Can you work these out from the model? Positions are in its coordinate system, mm. Face numbers are marked on the shaded views. A direction names the side the tool comes from. Round coordinates to 2 decimals unless told otherwise and drop trailing zeros. Loops run counter-clockwise (first coordinate to the right, second up) from the corner with the lowest first, then second, coordinate; pieces in that order, holes last. Notation, with made-up numbers: M 52.5,87 L 75.5,87 A15 ccw 75.5,116 Z; hole C 37,15.5 d11. An arc over 180 degrees is marked long. Return JSON: item names as keys, results as strings.
```python
from build123d import *

# Parameters (mm, degrees)
SKETCH_2_R      = 6.25
EXTRUDE_1_DEPTH = 15
SKETCH_3_W      = 12
SKETCH_3_H      = 18
EXTRUDE_2_DEPTH = 3
SKETCH_4_R      = 1.65
EXTRUDE_3_DEPTH = 5


with BuildPart() as part:
    # ｽｹｯﾁ2 → ﾎﾞｽ - 押し出し1 (new body)
    with BuildSketch(Plane.XY):
        Circle(SKETCH_2_R)
    extrude(amount=EXTRUDE_1_DEPTH)

    # ｽｹｯﾁ3 → ﾎﾞｽ - 押し出し2 (add)
    with BuildSketch(Plane.XY.offset(15)):
        Rectangle(SKETCH_3_W, SKETCH_3_H)
    extrude(amount=EXTRUDE_2_DEPTH)

    # ｽｹｯﾁ4 → ﾎﾞｽ - 押し出し3 (add, symmetric)
    with BuildSketch(Plane(origin=(0, 0, 0), x_dir=(0, 0, -1), z_dir=(1, 0, 0))):
        with BuildLine():
            Line((-18, 9), (-18, -9))
            Line((-18, -9), (-12, -9))
            ThreePointArc((-12, -9), (-65.69848481, 4.757359313), (-18, 33))
            Line((-18, 33), (-18, 9))
        make_face()
        with Locations((-36, 9)):
            Circle(SKETCH_4_R, mode=Mode.SUBTRACT)
    extrude(amount=EXTRUDE_3_DEPTH, both=True)


solid = part.part
```
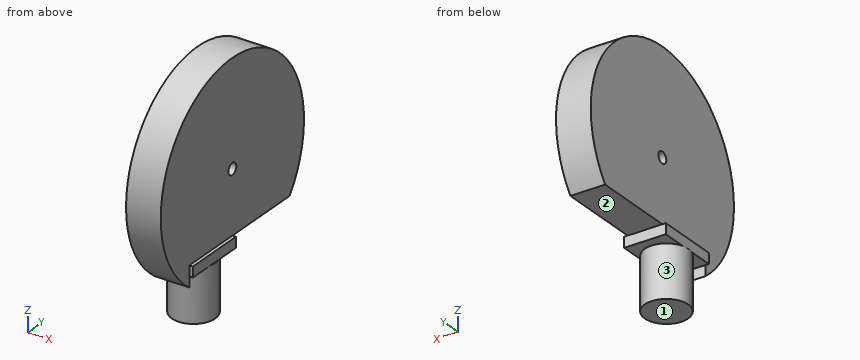
Q1. On a 3-axis mill with a long thin cutter (end or side, diameter ignored), from which of +Z, -Z, +X, -X, +Y, -Y can I reach the whole of each face in a straight line? I mean the marked faces 1, 2 and 3. Say none if no direction works.
Results:
{"face 1": "-Z, +X, -X, +Y, -Y", "face 2": "-Z, +X, -X, +Y", "face 3": "-Z"}
Q2. I'm going to push flat-ended pins straight in: pin 1 Ø1.5 at (x, y) = (-5, -6) entering from -Z; pin 2 Ø5.5 at (y, z) = (9, 36) entering from +X; pin 3 Ø1.5 at (x, z) = (0, 14) entering from +Y. Where does each tip first touch, or does it pass through?
Results:
{"pin 1": "stops at z = 15", "pin 2": "stops at x = 5", "pin 3": "stops at y = 6.25"}
Q3. Suppose I cut it at A-A, the plane x = 0. Please give me the cut outline in (y, z).
Results:
{"outline": "M -9,12 L -9,15 L -6.25,15 L -6.25,0 L 6.25,0 L 6.25,15 L 9,15 L 9,18 L 33,18 A30 ccw long Z; hole C 9,36 d3.3"}
Q4. Suppose I cut it at B-B, the plane z = 36. Please give me the cut outline in (x, y), plus the area to 3 significant figures.
Results:
{"outline": "M -5,-21 L 5,-21 L 5,7.35 L -5,7.35 Z; M -5,10.65 L 5,10.65 L 5,39 L -5,39 Z", "area": "567 mm2"}
Q5. If I drill on line 1 along Y through (x, z) = (-0.5, 36); line 2 along X through (y, z) = (-9.5, 48); line 3 along Y through (x, z) = (-0.25, 3) (3 decimals), over which ranges is the centre line in solid material (lowest first)?
Results:
{"line 1": "y = -21 to 7.35, 10.65 to 39", "line 2": "x = -5 to 5", "line 3": "y = -6.245 to 6.245"}
Q6. Suppose I cut it at C-C, the plane y = 0. Please give me the cut outline in (x, z), plus the area to 3 significant figures.
Results:
{"outline": "M -6.25,0 L 6.25,0 L 6.25,15 L 6,15 L 6,18 L 5,18 L 5,64.62 L -5,64.62 L -5,18 L -6,18 L -6,15 L -6.25,15 Z", "area": "690 mm2"}
Q7. Suppose I cut it at D-D, the plane z = 58. Please give me the cut outline in (x, y).
Results:
{"outline": "M -5,-11.4 L 5,-11.4 L 5,29.4 L -5,29.4 Z"}
